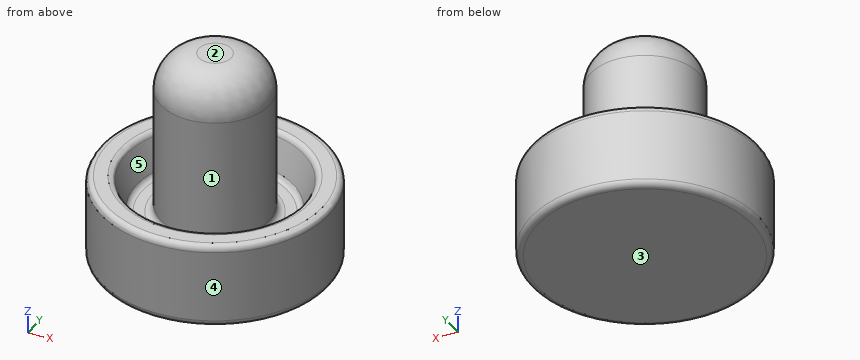
from build123d import *


with BuildPart() as f1:
    # F0 (on Right) → F1 (revolve)
    with BuildSketch(Plane.YZ):
        with BuildLine():
            Line((-21.429214, 0), (0, 0))
            Line((0, 0), (0, 42.777969))
            Line((0, 42.777969), (-3.227171, 42.777969))
            ThreePointArc((-3.227171, 42.777969), (-8.615325, 40.546123), (-10.847171, 35.157969))
            Line((-10.847171, 35.157969), (-10.847171, 10.86047))
            ThreePointArc((-10.847171, 10.86047), (-11.293541, 9.782839), (-12.371171, 9.33647))
            Line((-12.371171, 9.33647), (-14.463177, 9.33647))
            ThreePointArc((-14.463177, 9.33647), (-15.196262, 9.571237), (-15.65659, 10.188188))
            Line((-15.65659, 10.188188), (-17.671064, 16.048475))
            ThreePointArc((-17.671064, 16.048475), (-18.131391, 16.665426), (-18.864476, 16.900193))
            Line((-18.864476, 16.900193), (-21.429214, 16.900193))
            ThreePointArc((-21.429214, 16.900193), (-22.32155, 16.530575), (-22.691168, 15.638239))
            Line((-22.691168, 15.638239), (-22.691168, 1.261953))
            ThreePointArc((-22.691168, 1.261953), (-22.32155, 0.369618), (-21.429214, 0))
        make_face()
    revolve(axis=Axis((0, 0, 21.388984), (0, 0, 1)))


solid = f1.part
The listing builds one solid part. Answer for the finished solid, in the listing's coordinates (mm). Face numbers are marked on the shaded views. A direction names the side the tool comes from. Round coordinates to 2 decimals unless told otherwise and drop trailing zeros. Write each loop counter-clockwise with the first axis right and the second up, starting at its lowest first coordinate (ties: lowest second). Pieces come first, ordered by that corner, then holes. Notation, with made-up numbers: (15.25, -15.75) - (26.25, -15.75) arc R21 ccw to (26.25, 15.25) - close; hole circle Ø6 at (55.25, 23.25). An arc over 180 degrees is marked (long way). Use a Markdown table: item, result. Add a question column.
1. Flat-ended cylindrical pins translate along their axes: P1, Ø1.5, axis at y = 1.5, z = 25.5, coming from the -X side; P2, Ø21.5, axis at x = 8.5, y = 1.5, coming from the +Z side; P3, Ø1.5, axis at x = -5.5, z = 22, coming from the -Y side; P4, Ø5, axis at x = 12, y = 14.5, coming from the +Z side. Find the tip coordinate at first contact, or state that the pin passes through.
2. A tool of negligible diameter and unlimited length cuts with its end or side. For the marked faces 1 and 2, from which of +Z, -Z, +X, -X, +Y, -Y can it reach the whole face along a straight path? Write none if from no direction.
3. Consider line 1 (X direction, y = -8.5, z = 11); line 2 (Y direction, x = -10, z = 14.5); line 3 (X direction, y = 0, z = 7). Determine where each line is inside the solid, lowest interval first.
4. For a pull along Y with two mould halves and no side action, classify the marked faces 3, 4 and 5 as +Y half, -Y half, draft (parallel to the pull), parting line (faces both ways), or undercut.
5. The part is cut by section A-A (z = 7). Write down the section's boundary in (x, y), and give its area (3 significant figures).
6. The part is cut by section B-B (z = 20.5). Write down the section's boundary in (x, y), and give its area (3 significant figures).
Reported:
| question | item | result |
|---|---|---|
| 1 | P1 | x = -10.82 |
| 1 | P2 | z = 42.78 |
| 1 | P3 | y = -9.75 |
| 1 | P4 | z = 16.9 |
| 2 | face 1 | +Z |
| 2 | face 2 | +Z, +X, -X, +Y, -Y |
| 3 | line 1 | -21.04 to -13.48, -6.74 to 6.74, 13.48 to 21.04 |
| 3 | line 2 | -20.37 to -13.92, -4.2 to 4.2, 13.92 to 20.37 |
| 3 | line 3 | -22.69 to 22.69 |
| 4 | face 3 | draft |
| 4 | face 4 | parting line |
| 4 | face 5 | undercut |
| 5 | outline | circle Ø45.38 at (0, 0) |
| 5 | area | 1,620 mm^2 |
| 6 | outline | circle Ø21.69 at (0, 0) |
| 6 | area | 370 mm^2 |
